Can you work these out from the model? Positions are in its coordinate system, mm. A direction names the side the tool comes from. Give positions to 0.01 mm unless a question says otherwise; leave off trailing zeros. Order: outer loops, then holes, each group sorted by start corner. A loop starts at its lowest first (then second) coordinate and runs counter-clockwise, first axis right, second up.
```python
from build123d import *

# Parameters (mm, degrees)
F0_W     = 52
F0_H     = 40
F1_DEPTH = 40
F2_R     = 14
F3_DEPTH = 40.001
F4_R     = 2.25
F5_DEPTH = 17
F6_R     = 2.15
F7_DEPTH = 16
F8_SIZE  = 12
F9_SIZE  = 0.8


with BuildPart() as f1:
    # F0 (on Top) → F1 (new body)
    with BuildSketch(Plane.XY):
        Rectangle(F0_W, F0_H)
    extrude(amount=F1_DEPTH)

    # F2 (on face) → F3 (cut, through all)
    with BuildSketch(Plane.XZ.offset(20)):
        with Locations((0, 20)):
            Circle(F2_R)
    extrude(amount=-F3_DEPTH, mode=Mode.SUBTRACT)

    # F4 (on face) → F5 (cut)
    with BuildSketch(Plane.XY.offset(40)):
        with Locations((-20, 12)):
            Circle(F4_R)
        with Locations((-20, -12)):
            Circle(F4_R)
        with Locations((20, -12)):
            Circle(F4_R)
        with Locations((20, 12)):
            Circle(F4_R)
    extrude(amount=-F5_DEPTH, mode=Mode.SUBTRACT)

    # F6 (on face) → F7 (cut)
    with BuildSketch(Plane(origin=(0, 20, 0), x_dir=(-1, 0, 0), z_dir=(0, 1, 0))):
        with Locations((13.4350288425, 33.4350288425)):
            Circle(F6_R)
        with Locations((19, 20)):
            Circle(F6_R)
        with Locations((-13.4350288425, 33.4350288425)):
            Circle(F6_R)
        with Locations((-19, 20)):
            Circle(F6_R)
        with Locations((13.4350288425, 6.5649711575)):
            Circle(F6_R)
        with Locations((-13.4350288425, 6.5649711575)):
            Circle(F6_R)
    extrude(amount=-F7_DEPTH, mode=Mode.SUBTRACT)

    # F8
    f8_edges = [f1.edges().sort_by_distance(p)[0] for p in [
        (-26, 0, 0),
        (26, 0, 0),
    ]]
    chamfer(f8_edges, length=F8_SIZE)

    # F9
    f9_edges = [f1.edges().sort_by_distance(p)[0] for p in [
        (-26, 20, 26),
        (-20, 20, 6),
        (0, 20, 0),
        (20, 20, 6),
        (26, 20, 26),
        (0, 20, 40),
        (-26, -20, 26),
        (-20, -20, 6),
        (0, -20, 40),
        (0, -20, 0),
        (26, -20, 26),
        (20, -20, 6),
        (-14, -20, 20),
        (-14, 20, 20),
    ]]
    chamfer(f9_edges, length=F9_SIZE)


solid = f1.part
```
1) Which directions (+Z, -Z, +X, -X, +Y, -Y) give clear straight access to the entire face, cutting with the end or side of a thin tool? Please do faces 1 (the face through (19, 4, 20)), 2 (the face through (20, -12, 23)), 3 (the face through (0, -20, 37)).
2) I'm going to push flat-ended pins straight in: pin 1 Ø3.5 at (x, z) = (13.44, 33.44) entering from +Y; pin 2 Ø1.3 at (x, y) = (20.5, 12) entering from +Z; pin 3 Ø7 at (x, y) = (-20, 12) entering from -Z. Where does each tip first touch, or does it pass through?
3) We'd pull the mould along Z, two halves only. Please class faces 4 (the face through (22.146, -11.324, 31.619)), 5 (the face through (13, 4, 33)), 6 (the face through (20, 0, 6)): +Z half, -Z half, draft (parallel to the pull), parting line (faces both ways), or undercut.
4) Suppose I cut it at A-A (x = 0). Please give me the cut outline in (y, z), and give its area (3 significant figures).
5) Suppose I cut it at C-C (z = 32). Give the number of separate pieces and of enclosed holes in the cut face, and give its area (3 significant figures).
6) If I drill on line 1 (Y direction, x = -20, z = 29.5); line 2 (Z direction, x = 0, y = 3); line 3 (X direction, y = 13, z = 31.5), over which ranges is the centre line in solid material (lowest first)?
7) Suppose I cut it at B-B (y = -12). Please give me the cut outline in (x, z).
8) Suppose I cut it at D-D (y = -7). Please give me the cut outline in (x, z), and give its area (3 significant figures).
Results:
1. face 1: +Y
1. face 2: +Z
1. face 3: +Z, -Z, +X, -X, -Y
2. pin 1: stops at y = 4
2. pin 2: stops at z = 23
2. pin 3: stops at z = 2.5
3. face 4: draft
3. face 5: undercut
3. face 6: -Z half
4. outline: (-20, 0.8) - (-19.2, 0) - (19.2, 0) - (20, 0.8) - (20, 5.2) - (19.2, 6) - (-19.2, 6) - (-20, 5.2) - close; (-20, 34.8) - (-19.2, 34) - (19.2, 34) - (20, 34.8) - (20, 39.2) - (19.2, 40) - (-19.2, 40) - (-20, 39.2) - close
4. area: 477 mm2
5. separate pieces: 2
5. enclosed holes: 4
5. area: 1,330 mm2
6. line 1: y = -20 to -14.25, -9.75 to 9.75, 14.25 to 20
6. line 2: z = 0 to 6, 34 to 40
6. line 3: x = -26 to -22.02, -17.98 to -14.37, -12.5 to -7.98, 7.98 to 12.5, 14.37 to 17.98, 22.02 to 26
7. outline: (-26, 12) - (-14, 0) - (14, 0) - (26, 12) - (26, 40) - (22.25, 40) - (22.25, 23) - (17.75, 23) - (17.75, 40) - (-17.75, 40) - (-17.75, 23) - (-22.25, 23) - (-22.25, 40) - (-26, 40) - close; hole circle Ø28 at (0, 20)
8. outline: (-26, 12) - (-14, 0) - (14, 0) - (26, 12) - (26, 40) - (-26, 40) - close; hole circle Ø28 at (0, 20)
8. area: 1,320 mm2
